```python
from build123d import *

# Parameters (mm, degrees)
DODANIE_WYCI_GNI_CIE1_DEPTH = 5
WYTNIJ_WYCI_GNI_CIE1_REACH  = 87
SZKIC2_R                    = 2
SZKIC3_W                    = 30
SZKIC3_H                    = 30
DODANIE_WYCI_GNI_CIE2_DEPTH = 15
DODANIE_WYCI_GNI_CIE3_DEPTH = 5
DODANIE_WYCI_GNI_CIE4_DEPTH = 5
ZAOKR_GLENIE1_R             = 3
SZKIC6_W                    = 22
SZKIC6_H                    = 22
WYTNIJ_WYCI_GNI_CIE2_DEPTH  = 8.5


with BuildPart() as part:
    # Szkic1 → Dodanie-wyciągnięcie1 (new body)
    with BuildSketch(Plane.XY):
        Polygon((0, 0), (0, 60), (30, 60), (60, 30), (60, 0), align=None)
    extrude(amount=DODANIE_WYCI_GNI_CIE1_DEPTH)

    # Szkic2 → Wytnij-wyciągnięcie1 (cut, up to next)
    with BuildSketch(Plane(origin=(0, 0, 0), x_dir=(-1, 0, 0), z_dir=(0, 0, -1)), mode=Mode.PRIVATE) as wytnij_wyci_gni_cie1_sk1:
        with Locations((-45, 15)):
            Circle(SZKIC2_R)
    wytnij_wyci_gni_cie1_tool1 = extrude(wytnij_wyci_gni_cie1_sk1.sketch, amount=-WYTNIJ_WYCI_GNI_CIE1_REACH, mode=Mode.PRIVATE) & part.part
    # Szkic2 → Wytnij-wyciągnięcie1 (cut, up to next)
    with BuildSketch(Plane(origin=(0, 0, 0), x_dir=(-1, 0, 0), z_dir=(0, 0, -1)), mode=Mode.PRIVATE) as wytnij_wyci_gni_cie1_sk2:
        with Locations((-15, 45)):
            Circle(SZKIC2_R)
    wytnij_wyci_gni_cie1_tool2 = extrude(wytnij_wyci_gni_cie1_sk2.sketch, amount=-WYTNIJ_WYCI_GNI_CIE1_REACH, mode=Mode.PRIVATE) & part.part
    add(wytnij_wyci_gni_cie1_tool1.solids().sort_by_distance((45, 15, 0))[0], mode=Mode.SUBTRACT)
    add(wytnij_wyci_gni_cie1_tool2.solids().sort_by_distance((15, 45, 0))[0], mode=Mode.SUBTRACT)

    # Szkic3 → Dodanie-wyciągnięcie2 (add)
    with BuildSketch(Plane.XY.offset(5)):
        with Locations((15, 15)):
            Rectangle(SZKIC3_W, SZKIC3_H)
    extrude(amount=DODANIE_WYCI_GNI_CIE2_DEPTH)

    # Szkic4 → Dodanie-wyciągnięcie3 (add)
    with BuildSketch(Plane(origin=(0, 0, 0), x_dir=(-1, 0, 0), z_dir=(0, -1, 0))):
        Polygon((-30, -5), (-30, -20), (-60, -5), align=None)
    extrude(amount=-DODANIE_WYCI_GNI_CIE3_DEPTH)

    # Szkic5 → Dodanie-wyciągnięcie4 (add)
    with BuildSketch(Plane.ZY):
        Polygon((5, 30), (20, 30), (5, 60), align=None)
    extrude(amount=-DODANIE_WYCI_GNI_CIE4_DEPTH)

    # Zaokrąglenie1
    zaokr_glenie1_edges = [part.edges().sort_by_distance(p)[0] for p in [
        (0, 0, 10),
    ]]
    fillet(zaokr_glenie1_edges, radius=ZAOKR_GLENIE1_R)

    # Szkic6 → Wytnij-wyciągnięcie2 (cut)
    with BuildSketch(Plane.XY.offset(20)):
        with Locations((15, 15)):
            Rectangle(SZKIC6_W, SZKIC6_H)
    extrude(amount=-WYTNIJ_WYCI_GNI_CIE2_DEPTH, mode=Mode.SUBTRACT)


solid = part.part
```
Can you work these out from the model? Positions are in its coordinate system, mm. A direction names the side the tool comes from. Coordinates: 2 decimals unless noted, no trailing zeros. Order: outer loops, then holes, each group sorted by start corner. A loop starts at its lowest first (then second) coordinate and runs counter-clockwise, first axis right, second up. Notation, with made-up numbers: (40.5, 3.5) - (93.5, 3.5) arc R22 cw to (93.5, 22.5) - close; hole circle Ø11 at (31, 36). An arc over 180 degrees is marked (long way). Answer in a Markdown table with one row per item.
1. Suppose I cut it at B-B (y = 45). Please give me the cut outline in (x, z).
Reply:
| item | result |
|---|---|
| outline | (0, 0) - (13, 0) - (13, 5) - (5, 5) - (5, 12.5) - (0, 12.5) - close; (17, 0) - (45, 0) - (45, 5) - (17, 5) - close |
2. Suppose I cut it at D-D (z = 4.25). Please give me the cut outline in (x, y).
Reply:
| item | result |
|---|---|
| outline | (0, 3) arc R3 ccw to (3, 0) - (60, 0) - (60, 30) - (30, 60) - (0, 60) - close; hole circle Ø4 at (15, 45); hole circle Ø4 at (45, 15) |
3. If I drill on line 1 along Y through (x, z) = (15, 3.1); line 2 along X through (y, z) = (25, 17); line 3 along Z through (x, y) = (23, 16), over which ranges is the centre line in solid material (lowest first)?
Reply:
| item | result |
|---|---|
| line 1 | y = 0 to 43, 47 to 60 |
| line 2 | x = 0 to 4, 26 to 30 |
| line 3 | z = 0 to 11.5 |
4. For pin 1 (4 mm diameter, centred on y = 17, z = 10.5, fed in from +X); pin 2 (7 mm diameter, centred on x = 17, z = 15, fed in from +Y); pin 3 (2 mm diameter, centred on x = 41.5, y = 24, fed in from +Z); pin 4 (4.5 mm diameter, centred on y = 46.5, z = 15.5, fed in from +X), each with a flat end and sliding along its axis, tell me the tip position at first contact or that it passes through.
Reply:
| item | result |
|---|---|
| pin 1 | stops at x = 30 |
| pin 2 | stops at y = 30 |
| pin 3 | stops at z = 5 |
| pin 4 | passes through |
5. If we mould it in two halves opening along X, with no side actions, what happens to faces 4 (the flat face through (15, 15, 11.5)), 5 (the flat face through (45, 45, 2)), 6 (the flat face through (17, 30, 12))? For each: pulls with the +X half, pulls with the -X half, needs draft (parallel to the pull), parting line crosses it, or undercut.
Reply:
| item | result |
|---|---|
| face 4 | undercut |
| face 5 | pulls with the +X half |
| face 6 | needs draft |
6. Suppose I cut it at A-A (z = 15.5). Please give me the cut outline in (x, y), and give its area (3 significant figures).
Reply:
| item | result |
|---|---|
| outline | (0, 3) arc R3 ccw to (3, 0) - (39, 0) - (39, 5) - (30, 5) - (30, 30) - (5, 30) - (5, 39) - (0, 39) - close; hole (4, 4) - (26, 4) - (26, 26) - (4, 26) - close |
| area | 504 mm^2 |
7. For faces 1 (the flat face through (41, 5, 11)), 2 (the flat face through (44.8, 2.5, 12.6)), 3 (the flat face through (26, 15, 16)), which set-ups out of +Z, -Z, +X, -X, +Y, -Y let a thin tool reach every point of the face, with its end or its side?
Reply:
| item | result |
|---|---|
| face 1 | +Z, +X, +Y |
| face 2 | +Z, +X, +Y, -Y |
| face 3 | +Z |
